Design review of the part shown in the three views and the two pictorial views. Dimensions are in mm from the part's minimum x, y and z. A direction names the side the tool comes from. Give positions to 0.01 mm unless a question says otherwise; leave off trailing zeros. Loops run counter-clockwise (first coordinate to the right, second up) from the corner with the lowest first, then second, coordinate; pieces in that order, holes last. Notation, with made-up numbers: (55.5, -29.75) - (72.5, -29.75) arc R13 cw to (72.5, -11.75) - close; hole circle Ø1 at (57, 71). An arc over 180 degrees is marked (long way). Answer in a Markdown table with one row per item.
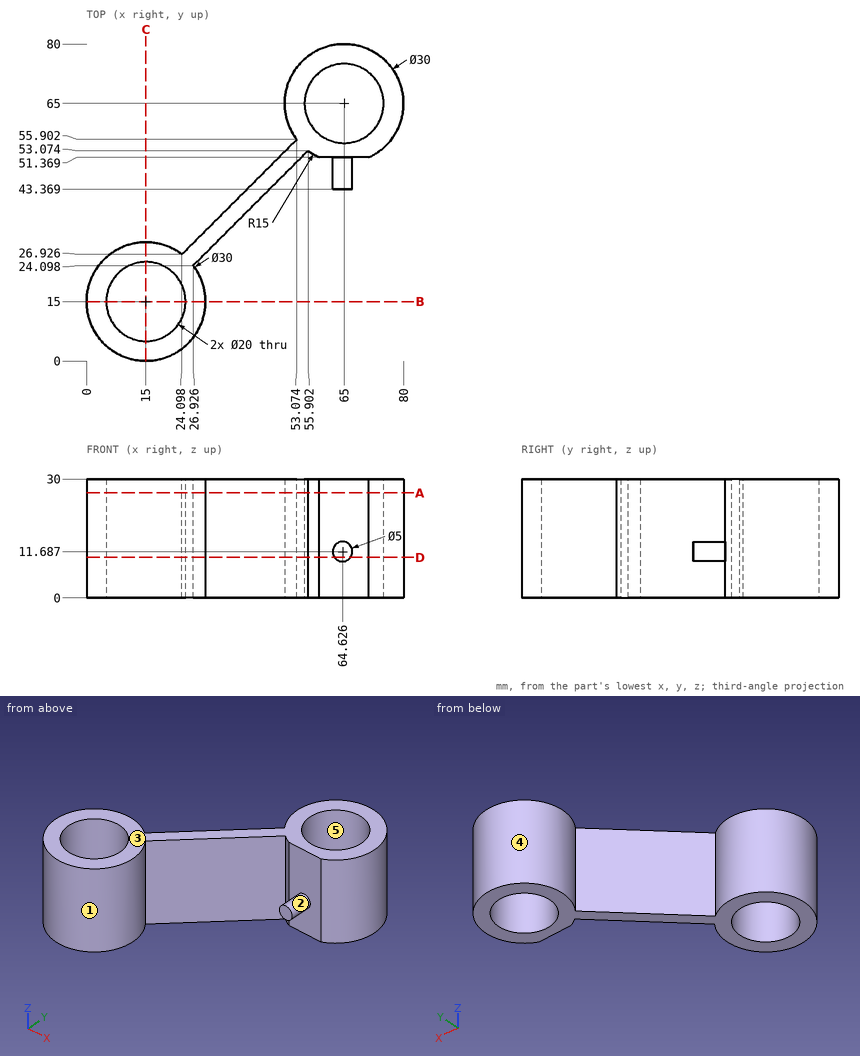
1. Clearance check with flat-ended pins moving along their axes: pin 1 (10 mm diameter, centred on y = 34, z = 5.5, fed in from +X); pin 2 (4 mm diameter, centred on y = 50.5, z = 6.5, fed in from +X); pin 3 (5 mm diameter, centred on x = 20, z = 7, fed in from -Y). State where each tip first meets the part, or that it passes through.
Values:
| item | result |
|---|---|
| pin 1 | stops at x = 41.83 |
| pin 2 | stops at x = 73.29 |
| pin 3 | stops at y = 0.21 |
2. For the marked faces 1 and 2, list the 3-axis set-ups (+Z, -Z, +X, -X, +Y, -Y) from which the entire face can be reached by the end or side of a thin tool; tool diameter is ignored.
Values:
| item | result |
|---|---|
| face 1 | +Z, -Z |
| face 2 | -Y |
3. We need section D-D, the plane z = 10.25. Give the boundary of the cut face in (x, y).
Values:
| item | result |
|---|---|
| outline | (24.1, 26.93) arc R15 ccw (long way) to (26.93, 24.1) - (55.9, 53.07) arc R15 ccw to (58.74, 51.37) - (62.58, 51.37) - (62.58, 43.37) - (66.67, 43.37) - (66.67, 51.37) - (71.26, 51.37) arc R15 ccw (long way) to (53.07, 55.9) - close; hole circle Ø20 at (15, 15); hole circle Ø20 at (65, 65) |
4. Mouldability with a two-part tool opening along X and no side actions: class the marked faces 3, 4 and 5 as released by +X, released by -X, zero draft, split by the parting line, or undercut.
Values:
| item | result |
|---|---|
| face 3 | zero draft |
| face 4 | split by the parting line |
| face 5 | undercut |
5. Wall thickness on line 1 (X direction, y = 72.5, z = 10.25) (1 decimal); line 2 (Y direction, x = 65, z = 20.5); line 3 (Y direction, x = 15, z = 6): over which ranges is each line inside the solid? List them lowest first. Write a range as [from, to].
Values:
| item | result |
|---|---|
| line 1 | x = [52, 58.4], [71.6, 78] |
| line 2 | y = [51.37, 55], [75, 80] |
| line 3 | y = [0, 5], [25, 30] |
6. We need section A-A, the plane z = 26.5. Give the boundary of the cut face in (x, y), and give its area (3 significant figures).
Values:
| item | result |
|---|---|
| outline | (24.1, 26.93) arc R15 ccw (long way) to (26.93, 24.1) - (55.9, 53.07) arc R15 ccw to (58.74, 51.37) - (71.26, 51.37) arc R15 ccw (long way) to (53.07, 55.9) - close; hole circle Ø20 at (15, 15); hole circle Ø20 at (65, 65) |
| area | 937 mm^2 |
7. We need section B-B, the plane y = 15. Give the boundary of the cut face in (x, z), and give its area (3 significant figures).
Values:
| item | result |
|---|---|
| outline | (0, 0) - (5, 0) - (5, 30) - (0, 30) - close; (25, 0) - (30, 0) - (30, 30) - (25, 30) - close |
| area | 300 mm^2 |
